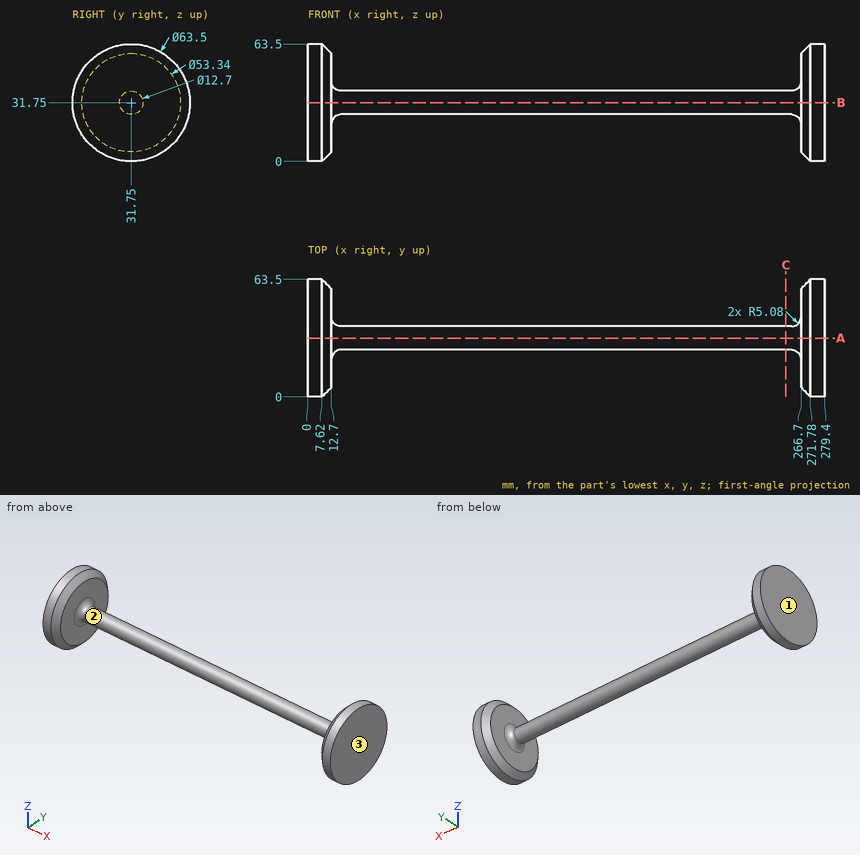
Part print with two shaded views. Sizes in mm from the minimum x, y, z corner. Round coordinates to 2 decimals unless told otherwise and drop trailing zeros. Order: outer loops, then holes, each group sorted by start corner. A loop starts at its lowest first (then second) coordinate and runs counter-clockwise, first axis right, second up. Notation, with made-up numbers: (37.25, -32.75) - (77.25, -32.75) arc R13 cw to (77.25, -18.75) - close; hole circle Ø7 at (88.5, 55.5). An arc over 180 degrees is marked (long way). Answer in a Markdown table with one row per item. Add a question column.
(1) Band-saw the part on C-C on x = 258.5. List the corners of the cut face in (y, z).
(2) Mould opens along X. For the marked faces 1, 2 and 3 say: +X half, -X half, draft (parallel to the pull), parting line (faces both ways), or undercut.
(3) Drop flat-ended pins along their axis: pin 1 Ø1.5 at (x, z) = (47.5, 27) entering from -Y; pin 2 Ø3 at (x, z) = (150.5, 30) entering from +Y; pin 3 Ø10 at (x, z) = (205.5, 23) entering from -Y. Give the stop position or say it passes through.
(4) Probe L1, parallel to X at y = 21, z = 49; L2, parallel to X at y = 19.5, z = 59; L3, parallel to Z at x = 219, y = 32. List the from-to ranges inside material, lowest first. Write a range as [from, to].
(5) Band-saw the part on A-A on y = 31.75. List the corners of the cut face in (x, z), and give its area (3 significant figures).
Data:
| question | item | result |
|---|---|---|
| 1 | outline | circle Ø12.7 at (31.75, 31.75) |
| 2 | face 1 | -X half |
| 2 | face 2 | undercut |
| 2 | face 3 | +X half |
| 3 | pin 1 | stops at y = 26.82 |
| 3 | pin 2 | stops at y = 38.1 |
| 3 | pin 3 | stops at y = 26.63 |
| 4 | L1 | x = [0, 12.7], [266.7, 279.4] |
| 4 | L2 | x = [0, 9.49], [269.91, 279.4] |
| 4 | L3 | z = [25.4, 38.1] |
| 5 | outline | (0, 0) - (7.62, 0) - (12.7, 5.08) - (12.7, 20.32) arc R5.08 cw to (17.78, 25.4) - (261.62, 25.4) arc R5.08 cw to (266.7, 20.32) - (266.7, 5.08) - (271.78, 0) - (279.4, 0) - (279.4, 63.5) - (271.78, 63.5) - (266.7, 58.42) - (266.7, 43.18) arc R5.08 cw to (261.62, 38.1) - (17.78, 38.1) arc R5.08 cw to (12.7, 43.18) - (12.7, 58.42) - (7.62, 63.5) - (0, 63.5) - close |
| 5 | area | 4,810 mm^2 |
